Verification items for the finished model (mm, model axes). Face numbers are marked on the shaded views. A direction names the side the tool comes from. Round coordinates to 2 decimals unless told otherwise and drop trailing zeros. Order: outer loops, then holes, each group sorted by start corner. A loop starts at its lowest first (then second) coordinate and runs counter-clockwise, first axis right, second up. Notation, with made-up numbers: (26.5, 76) -> (49.5, 76) arc R20 ccw to (49.5, 96) -> close; hole circle Ø11 at (8, -31.75). An arc over 180 degrees is marked (long way). Return JSON: item names as keys, results as strings. Group by question number.
1) Depth check by flat-ended pin: pin 1 (3 mm diameter, centred on x = 2, y = 2, fed in from +Z); pin 2 (1.9 mm diameter, centred on y = 6.5, z = -5.5, fed in from -X); pin 3 (1 mm diameter, centred on x = -3, y = 3, fed in from +Z); pin 4 (6 mm diameter, centred on x = -2, z = -2, fed in from +Y). Enter the tip coordinate at first touch or a pass-through.
2) Tool access check on the marked faces 4, 5 and 6. Record the directions out of +Z, -Z, +X, -X, +Y, -Y that give a thin tool (end or side, any length) a straight path to the whole face; none if there is none.
3) Section check B-B on z = 0. Enter the section's corners in (x, y), plus the area to 3 significant figures.
4) Section check A-A on y = 5. Enter the section's corners in (x, z).
5) Scan lines: L1, parallel to X at y = 4, z = 2.5; L2, parallel to Y at x = 0.25, z = -3.5; L3, parallel to X at y = 3.75, z = 2.25. Record each from-to range of solid material in increasing order.
6) Draft check along X on the marked faces 1, 2 and 3. Enter one of: pulls with the +X half, pulls with the -X half, needs draft (parallel to the pull), parting line crosses it, or undercut.
```python
from build123d import *

# Parameters (mm, degrees)
SKETCH1_R           = 5
BOSS_EXTRUDE1_DEPTH = 1.6
BOSS_EXTRUDE2_DEPTH = 8.1
CIRPATTERN3_COUNT   = 3
CUT_EXTRUDE2_DEPTH  = 13.097652285
CUT_EXTRUDE3_DEPTH  = 13.164834188
CUT_EXTRUDE4_DEPTH  = 12.917406966
FILLET1_R           = 1.2


with BuildPart() as part:
    # Sketch1 → Boss-Extrude1 (new body)
    with BuildSketch(Plane(origin=(0, 0, 0), x_dir=(1, 0, 0), z_dir=(0, 1, 0))):
        with Locations(Location((0, 0, 0), (0, 0, 270))):
            Circle(SKETCH1_R)
    extrude(amount=BOSS_EXTRUDE1_DEPTH)

    # Sketch2 → Boss-Extrude2 (add)
    with BuildSketch(Plane(origin=(0, 1.6, 0), x_dir=(1, 0, 0), z_dir=(0, 1, 0))):
        with BuildLine():
            Line((-1.2, 4.85386444), (-1.2, 3.815756806))
            ThreePointArc((-1.2, 3.815756806), (0, 4), (1.2, 3.815756806))
            Line((1.2, 3.815756806), (1.2, 4.85386444))
            ThreePointArc((1.2, 4.85386444), (0, 5), (-1.2, 4.85386444))
        make_face()
    boss_extrude2 = extrude(amount=BOSS_EXTRUDE2_DEPTH)

    # CirPattern3: Boss-Extrude2 ×3 about axis
    cirpattern3_axis = Axis((0, 0, 0), (0, 1, 0))
    for i in range(1, CIRPATTERN3_COUNT):
        add(boss_extrude2.rotate(cirpattern3_axis, i * 360 / CIRPATTERN3_COUNT))

    # Sweep3: sweep along a path in Sketch6
    with BuildLine(Plane(origin=(0, 9.7, 0), x_dir=(1, 0, 0), z_dir=(0, 1, 0))) as sweep3_path:
        CenterArc((0, 0), 5, 0, 360)
    # Sketch3 → Sweep3 (sweep)
    with BuildSketch(Plane(origin=(0, 0, 0), x_dir=(0, 0, -1), z_dir=(1, 0, 0))):
        Polygon((5.05386444, 9.7), (6.35386444, 8.2), (4.85386444, 8.2), (4.85386444, 9.7), align=None)
    sweep(path=sweep3_path.line)

    # Sketch7 → Cut-Extrude2 (cut, through all)
    with BuildSketch(Plane(origin=(0, 1.6, 0), x_dir=(1, 0, 0), z_dir=(0, 1, 0))):
        with BuildLine():
            Line((-3.904542328, -0.868647918), (-4.803569911, -1.387701735))
            ThreePointArc((-4.803569911, -1.387701735), (-4.330127019, 2.5), (-1.2, 4.85386444))
            Line((-1.2, 4.85386444), (-1.2, 3.815756806))
            ThreePointArc((-1.2, 3.815756806), (0, 4), (1.2, 3.815756806))
            Line((1.2, 3.815756806), (1.2, 4.85386444))
            ThreePointArc((1.2, 4.85386444), (4.330127019, 2.5), (4.803569911, -1.387701735))
            Line((4.803569911, -1.387701735), (3.904542328, -0.868647918))
            ThreePointArc((3.904542328, -0.868647918), (3.464101615, -2), (2.704542328, -2.947108887))
            Line((2.704542328, -2.947108887), (3.603569911, -3.466162704))
            ThreePointArc((3.603569911, -3.466162704), (0, -5), (-3.603569911, -3.466162704))
            Line((-3.603569911, -3.466162704), (-2.704542328, -2.947108887))
            ThreePointArc((-2.704542328, -2.947108887), (-3.464101615, -2), (-3.904542328, -0.868647918))
        make_face()
    extrude(amount=CUT_EXTRUDE2_DEPTH, mode=Mode.SUBTRACT)

    # Sketch8 → Cut-Extrude3 (cut, through all)
    with BuildSketch(Plane.XZ.offset(-8.2)):
        with BuildLine():
            Line((-3.603569911, 3.466162704), (-4.803581682, 4.158989823))
            ThreePointArc((-4.803581682, 4.158989823), (0, 6.35386444), (4.803581682, 4.158989823))
            Line((4.803581682, 4.158989823), (3.603569911, 3.466162704))
            ThreePointArc((3.603569911, 3.466162704), (0, 5), (-3.603569911, 3.466162704))
        make_face()
        with BuildLine():
            Line((-6.003581682, 2.080528854), (-4.803569911, 1.387701735))
            ThreePointArc((-4.803569911, 1.387701735), (-4.330127019, -2.5), (-1.2, -4.85386444))
            Line((-1.2, -4.85386444), (-1.2, -6.239518677))
            ThreePointArc((-1.2, -6.239518677), (-5.502608017, -3.17693222), (-6.003581682, 2.080528854))
        make_face()
        with BuildLine():
            Line((1.2, -6.239518677), (1.2, -4.85386444))
            ThreePointArc((1.2, -4.85386444), (4.330127019, -2.5), (4.803569911, 1.387701735))
            Line((4.803569911, 1.387701735), (6.003581682, 2.080528854))
            ThreePointArc((6.003581682, 2.080528854), (5.502608017, -3.17693222), (1.2, -6.239518677))
        make_face()
    extrude(amount=-CUT_EXTRUDE3_DEPTH, mode=Mode.SUBTRACT)

    # Sketch9 → Cut-Extrude4 (cut, through all)
    with BuildSketch(Plane(origin=(0, 1.6, 0), x_dir=(1, 0, 0), z_dir=(0, 1, 0))):
        with BuildLine():
            Line((1.9, -3.15), (1.9, 1.25))
            ThreePointArc((1.9, 1.25), (0, 3.15), (-1.9, 1.25))
            Line((-1.9, 1.25), (-1.9, -3.15))
            Line((-1.9, -3.15), (1.9, -3.15))
        make_face()
    extrude(amount=-CUT_EXTRUDE4_DEPTH, mode=Mode.SUBTRACT)

    # Fillet1
    fillet1_edges = [part.edges().sort_by_distance(p)[0] for p in [
        (1.9, 0.8, 3.15),
        (-1.9, 0.8, 3.15),
    ]]
    fillet(fillet1_edges, radius=FILLET1_R)


solid = part.part
```
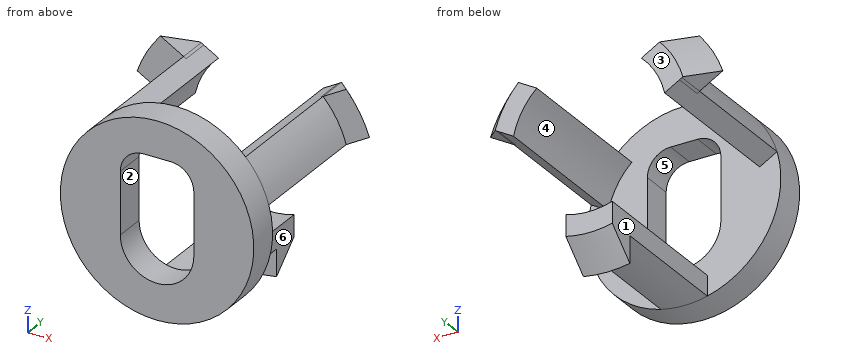
Check result:
{
 "1": {"pin 1": "z = 4.97", "pin 2": "x = -1.2", "pin 3": "z = 3.41", "pin 4": "y = 9.7"},
 "2": {"face 4": "-Z, +Y", "face 5": "+Y, -Y", "face 6": "+Z, -Z, +X, +Y"},
 "3": {"outline": "(-5, 0) -> (-1.9, 0) -> (-1.9, 1.6) -> (-5, 1.6) -> close; (1.9, 0) -> (5, 0) -> (5, 1.6) -> (1.9, 1.6) -> close", "area": "9.92 mm^2"},
 "4": {"outline": "(-4.8, 1.39) -> (-3.9, 0.87) arc R4 cw to (-2.7, 2.95) -> (-3.6, 3.47) arc R5 ccw to start; (-1.2, -4.85) arc R5 ccw to (1.2, -4.85) -> (1.2, -3.82) arc R4 cw to (-1.2, -3.82) -> close; (2.7, 2.95) arc R4 cw to (3.9, 0.87) -> (4.8, 1.39) arc R5 ccw to (3.6, 3.47) -> close"},
 "5": {"L1": "-4.33 to -3.12, 3.12 to 4.33", "L2": "0 to 1.6", "L3": "-4.47 to -3.31, 3.31 to 4.47"},
 "6": {"face 1": "pulls with the -X half", "face 2": "undercut", "face 3": "needs draft"}
}
